Solid Edge part; units mm, degrees
sketch "Sketch1" plane through (0, 0, 0) normal (0, -1, 0) x (1, 0, 0)
  circle A0 centre (0, 0) radius 16.5
  circle A1 centre (0, 0) radius 13.5
extrude "Protrusion1" add sketch "Sketch1" against normal blind 1.5
sketch "Sketch2" plane through (0, 1.5, 0) normal (0, 1, 0) x (1, 0, 0)
  line L0 (-1.8277, 13.3757) -> (-1.8277, 16.3985)
  arc A0 (1.8277, 16.3985) -> (-1.8277, 16.3985) centre (0, 0) ccw
  line L1 (1.8277, 16.3985) -> (1.8277, 13.3757)
  arc A1 (1.8277, 13.3757) -> (-1.8277, 13.3757) centre (0, 0) ccw
extrude "ExtrudedCutout_1" cut sketch "Sketch2" against normal blind 12.4809
fillet "Round_1" radius 0.5 4 edges at (-1.8277, 0.75, -13.3757) (-1.8277, 0.75, -16.3985) (1.8277, 0.75, -16.3985) (1.8277, 0.75, -13.3757)
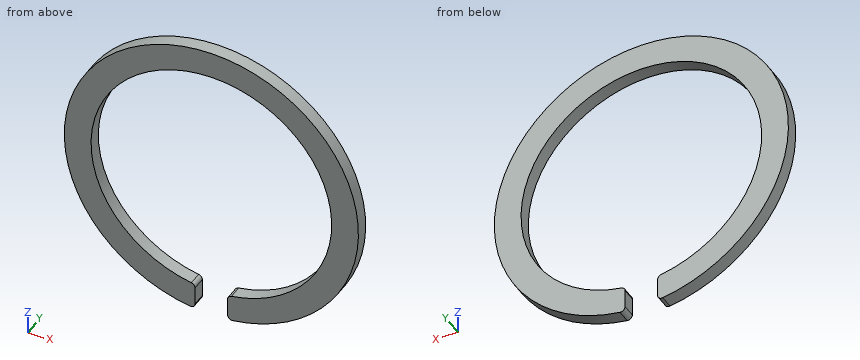
Here's how the part is built. I have some questions about the finished solid (model axes, mm). Round coordinates to 2 decimals unless told otherwise and drop trailing zeros. Order: outer loops, then holes, each group sorted by start corner. A loop starts at its lowest first (then second) coordinate and runs counter-clockwise, first axis right, second up. Notation, with made-up numbers: M 59,15 L 78,15 A6 cw 78,23 Z; hole C 33.25,19.5 d9. An arc over 180 degrees is marked long. Return JSON: item names as keys, results as strings. Group by question number.
1. If we section it at C-C on y = 1: List the corners of the cut face in (x, z) for me.
2. If we section it at D-D on x = 0: List the corners of the cut face in (y, z) for me.
3. If we section it at B-B on x = 6: List the corners of the cut face in (y, z) for me.
4. Please list where these lines run through material, in increasing order: probe 1 along X at (y, z) = (1, 0); probe 2 along Z at (x, y) = (6.5, 1.3); probe 3 along Z at (x, y) = (0, 0.75).
5. I'm going to push flat-ended pins straight in: pin 1 Ø12 at (x, z) = (0, 1.5) entering from -Y; pin 2 Ø0.8 at (y, z) = (1, -15) entering from +X. Where does each tip first touch, or does it pass through?
6. If we section it at A-A on z = 0: List the corners of the cut face in (x, y) for me, then the cut area to 3 significant figures.
Reply:
{
 "1": {"outline": "M -2.4,-16.32 A0.5 ccw -1.83,-15.83 L -1.83,-13.81 A0.5 ccw -2.24,-13.31 A13.5 cw long 2.24,-13.31 A0.5 ccw 1.83,-13.81 L 1.83,-15.83 A0.5 ccw 2.4,-16.32 A16.5 ccw long Z"},
 "2": {"outline": "M 0,13.5 L 1.5,13.5 L 1.5,16.5 L 0,16.5 Z"},
 "3": {"outline": "M 0,-15.37 L 1.5,-15.37 L 1.5,-12.09 L 0,-12.09 Z; M 0,12.09 L 1.5,12.09 L 1.5,15.37 L 0,15.37 Z"},
 "4": {"probe 1": "-16.5 to -13.5, 13.5 to 16.5", "probe 2": "-15.17 to -11.83, 11.83 to 15.17", "probe 3": "13.5 to 16.5"},
 "5": {"pin 1": "through", "pin 2": "x = 7.69"},
 "6": {"outline": "M -16.5,0 L -13.5,0 L -13.5,1.5 L -16.5,1.5 Z; M 13.5,0 L 16.5,0 L 16.5,1.5 L 13.5,1.5 Z", "area": "9.00 mm^2"}
}
